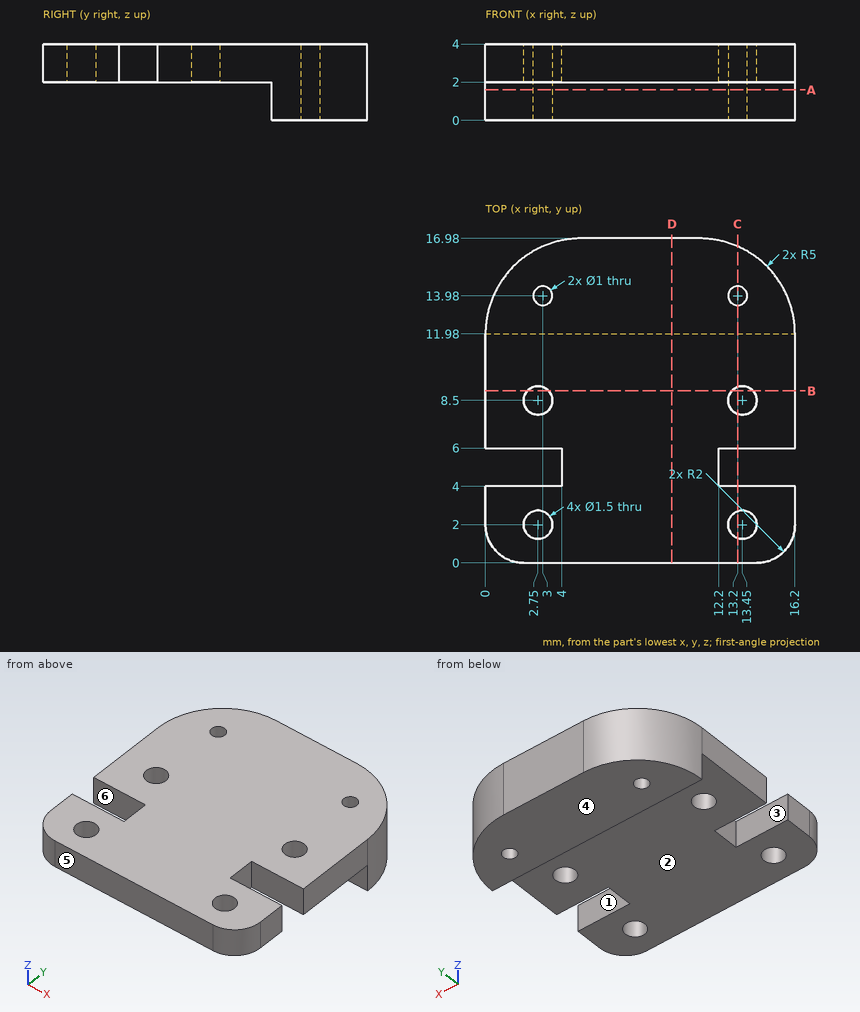
The figure shows three views and two pictorial views of one solid part (mm, origin at its lowest corner). Answer the questions. A direction names the side the tool comes from. Round coordinates to 2 decimals unless told otherwise and drop trailing zeros. Order: outer loops, then holes, each group sorted by start corner. A loop starts at its lowest first (then second) coordinate and runs counter-clockwise, first axis right, second up.
Q1. Given pin 1 Ø2 at (x, y) = (13.45, 8.5) entering from -Z; pin 2 Ø0.6 at (x, z) = (2, 3) entering from +Y; pin 3 Ø0.9 at (x, y) = (2.75, 2) entering from -Z; pin 4 Ø1.6 at (x, z) = (4.5, 0.5) entering from -Y, each flat-ended and moving along its own axis, determine where each tip first touches the part or whether it passes through.
Solution:
pin 1: stops at z = 2
pin 2: stops at y = 16.19
pin 3: passes through
pin 4: stops at y = 11.98
Q2. A cutting plane is placed at A-A, the plane z = 1.6. Determine the outline of the cut face in (x, y), then the cut area to 3 significant figures.
Solution:
outline: (0, 11.98) - (16.2, 11.98) arc R5 ccw to (11.2, 16.98) - (5, 16.98) arc R5 ccw to start; hole circle Ø1 at (3, 13.98); hole circle Ø1 at (13.2, 13.98)
area: 68.7 mm2
Q3. Find the intervals of material crossed by line 1 along X through (y, z) = (8.5, 2.55); line 2 along Y through (x, z) = (13.2, 2.7); line 3 along Z through (x, y) = (11, 8.5), in increasing order.
Solution:
line 1: x = 0 to 2, 3.5 to 12.7, 14.2 to 16.2
line 2: y = 0 to 1.29, 2.71 to 4, 6 to 7.79, 9.21 to 13.48, 14.48 to 16.56
line 3: z = 2 to 4
Q4. The mould has two halves that part along Y. Classify the marked faces 4, 5 and 6: pulls with the +Y half, pulls with the -Y half, needs draft (parallel to the pull), parting line crosses it, or undercut.
Solution:
face 4: needs draft
face 5: pulls with the -Y half
face 6: undercut
Q5. A tool of negligible diameter and unlimited length cuts with its end or side. For the marked faces 1, 2 and 3, from which of +Z, -Z, +X, -X, +Y, -Y can it reach the whole face along a straight path? Write none if from no direction.
Solution:
face 1: +Z, -Z, +X
face 2: -Z, +X, -X, -Y
face 3: +Z, -Z, -X
Q6. A cutting plane is placed at D-D, the plane x = 9.75. Determine the outline of the cut face in (y, z).
Solution:
outline: (0, 2) - (11.98, 2) - (11.98, 0) - (16.98, 0) - (16.98, 4) - (0, 4) - close
Q7. A cutting plane is placed at C-C, the plane x = 13.2. Determine the outline of the cut face in (y, z), then the cut area to 3 significant figures.
Solution:
outline: (0, 2) - (1.29, 2) - (1.29, 4) - (0, 4) - close; (2.71, 2) - (4, 2) - (4, 4) - (2.71, 4) - close; (6, 2) - (7.79, 2) - (7.79, 4) - (6, 4) - close; (9.21, 2) - (11.98, 2) - (11.98, 0) - (13.48, 0) - (13.48, 4) - (9.21, 4) - close; (14.48, 0) - (16.56, 0) - (16.56, 4) - (14.48, 4) - close
area: 28.6 mm2
Q8. A cutting plane is placed at B-B, the plane y = 9. Determine the outline of the cut face in (x, z), then the cut area to 3 significant figures.
Solution:
outline: (0, 2) - (2.19, 2) - (2.19, 4) - (0, 4) - close; (3.31, 2) - (12.89, 2) - (12.89, 4) - (3.31, 4) - close; (14.01, 2) - (16.2, 2) - (16.2, 4) - (14.01, 4) - close
area: 27.9 mm2
